```python
from build123d import *

# Parameters (mm, degrees)
SKETCH3_R          = 0.5
CUT_EXTRUDE1_DEPTH = 10
FILLET1_R          = 0.5
CHAMFER1_SIZE      = 0.2
SKETCH4_W          = 1
SKETCH4_H          = 12.5
SKETCH4_W_2        = 12.5
SKETCH4_H_2        = 1
CUT_EXTRUDE2_DEPTH = 4


with BuildPart() as part:
    # Sketch2 → Revolve1 (revolve)
    with BuildSketch(Plane(origin=(0, 0, 0), x_dir=(0, 0, -1), z_dir=(1, 0, 0)), mode=Mode.PRIVATE) as revolve1_sk:
        Polygon((0, 0), (0, 7.25), (1, 7.25), (1, 6.1), (5, 6.1), (5, 5.1), (1, 5.1), (1, 0), align=None)
    revolve(revolve1_sk.sketch.rotate(Axis((0, 0, 0), (0, 0, -1)), 90), axis=Axis((0, 0, 0), (0, 0, -1)))

    # Sketch3 → Cut-Extrude1 (cut)
    with BuildSketch(Plane.XY):
        with Locations((-1.425, 1.425)):
            Circle(SKETCH3_R)
        with Locations((1.425, 1.425)):
            Circle(SKETCH3_R)
        with Locations((0, 1.425)):
            Circle(SKETCH3_R)
        with Locations((1.425, 0)):
            Circle(SKETCH3_R)
        with Locations((1.425, -1.425)):
            Circle(SKETCH3_R)
        with Locations((0, -1.425)):
            Circle(SKETCH3_R)
        with Locations((-1.425, -1.425)):
            Circle(SKETCH3_R)
        with Locations((-1.425, 0)):
            Circle(SKETCH3_R)
        with Locations((-2.925, 2.925)):
            Circle(SKETCH3_R)
        with Locations((0, 2.925)):
            Circle(SKETCH3_R)
        with Locations((2.925, 2.925)):
            Circle(SKETCH3_R)
        with Locations((2.925, 0)):
            Circle(SKETCH3_R)
        with Locations((2.925, -2.925)):
            Circle(SKETCH3_R)
        with Locations((0, -2.925)):
            Circle(SKETCH3_R)
        with Locations((-2.925, -2.925)):
            Circle(SKETCH3_R)
        with Locations((-2.925, 0)):
            Circle(SKETCH3_R)
        with Locations((-1.425, 2.925)):
            Circle(SKETCH3_R)
        with Locations((1.425, 2.925)):
            Circle(SKETCH3_R)
        with Locations((2.925, 1.425)):
            Circle(SKETCH3_R)
        with Locations((2.925, -1.425)):
            Circle(SKETCH3_R)
        with Locations((1.425, -2.925)):
            Circle(SKETCH3_R)
        with Locations((-1.425, -2.925)):
            Circle(SKETCH3_R)
        with Locations((-2.925, -1.425)):
            Circle(SKETCH3_R)
        with Locations((-2.925, 1.425)):
            Circle(SKETCH3_R)
        with Locations((-1.425, 4.225)):
            Circle(SKETCH3_R)
        with Locations((0, 4.225)):
            Circle(SKETCH3_R)
        with Locations((1.425, 4.225)):
            Circle(SKETCH3_R)
        with Locations((4.225, 1.425)):
            Circle(SKETCH3_R)
        with Locations((4.225, 0)):
            Circle(SKETCH3_R)
        with Locations((4.225, -1.425)):
            Circle(SKETCH3_R)
        with Locations((1.425, -4.225)):
            Circle(SKETCH3_R)
        with Locations((0, -4.225)):
            Circle(SKETCH3_R)
        with Locations((-1.425, -4.225)):
            Circle(SKETCH3_R)
        with Locations((-4.225, -1.425)):
            Circle(SKETCH3_R)
        with Locations((-4.225, 0)):
            Circle(SKETCH3_R)
        with Locations((-4.225, 1.425)):
            Circle(SKETCH3_R)
        Circle(SKETCH3_R)
    extrude(amount=-CUT_EXTRUDE1_DEPTH, mode=Mode.SUBTRACT)

    # Fillet1
    fillet1_edges = [part.edges().sort_by_distance(p)[0] for p in [
        (-6.1, 0, -5),
        (-7.25, 0, 0),
    ]]
    fillet(fillet1_edges, radius=FILLET1_R)

    # Chamfer1
    chamfer1_edges = [part.edges().sort_by_distance(p)[0] for p in [
        (-5.1, 0, -5),
    ]]
    chamfer(chamfer1_edges, length=CHAMFER1_SIZE)

    # Sketch4 → Cut-Extrude2 (cut)
    with BuildSketch(Plane(origin=(0, 0, -5), x_dir=(-1, 0, 0), z_dir=(0, 0, -1))):
        Rectangle(SKETCH4_W, SKETCH4_H)
        Rectangle(SKETCH4_W_2, SKETCH4_H_2)
    extrude(amount=-CUT_EXTRUDE2_DEPTH, mode=Mode.SUBTRACT)


solid = part.part
```
Design review of the part built by this model. Coordinates are the model's own, in mm. A direction names the side the tool comes from. Give positions to 0.01 mm unless a question says otherwise; leave off trailing zeros. Order: outer loops, then holes, each group sorted by start corner. A loop starts at its lowest first (then second) coordinate and runs counter-clockwise, first axis right, second up. Notation, with made-up numbers: (7.5, 72.5) - (62.5, 72.5) arc R29 cw to (62.5, 92.5) - close; hole circle Ø8 at (74, 28). An arc over 180 degrees is marked (long way). Use a Markdown table: item, result. Add a question column.
(1) Clearance check with flat-ended pins moving along their axes: P1, Ø1.1, axis at x = 6, z = -3.5, coming from the +Y side; P2, Ø1.5, axis at y = 2, z = -2, coming from the +X side; P3, Ø1.1, axis at y = 5.5, z = -2, coming from the +X side. State where each tip first meets the part, or that it passes through.
(2) Wall thickness on probe 1 along X at (y, z) = (-2.75, -0.4); probe 2 along X at (y, z) = (-1, -4.25); probe 3 along X at (y, z) = (-1.25, -1.55): over which ranges is each line inside the solid? List them lowest first. Write a range as [from, to].
(3) Machinability: for faces 1 (the face through (5.6, 0.5, -3)), 2 (the face through (3.16, -0.44, -0.49)), which of the approach directions +Z, -Z, +X, -X, +Y, -Y give a long, thin tool a straight path to every point of the face, cutting with its end or side? Answer none if there is none.
(4) Add section A-A on x = 0. Give the number of separate pieces and of enclosed holes in the cut face, then the cut area to 3 significant figures.
(5) Add section C-C on z = -3.85. Give the boundary of the cut face in (x, y).
Report:
| question | item | result |
|---|---|---|
| 1 | P1 | stops at y = 2.74 |
| 1 | P2 | stops at x = 5.97 |
| 1 | P3 | stops at x = 3.56 |
| 2 | probe 1 | x = [-6.7, -3.39], [-2.46, -1.89], [-0.96, -0.47], [0.47, 0.96], [1.89, 2.46], [3.39, 6.7] |
| 2 | probe 2 | x = [-6.02, -5], [5, 6.02] |
| 2 | probe 3 | x = [-5.97, -4.94], [4.94, 5.97] |
| 3 | face 1 | -Z, +X, -X |
| 3 | face 2 | +Z, -Z |
| 4 | separate pieces | 8 |
| 4 | enclosed holes | 0 |
| 4 | area | 7.39 mm² |
| 5 | outline | (-6.08, -0.5) arc R6.1 ccw to (-0.5, -6.08) - (-0.5, -5.08) arc R5.1 cw to (-5.08, -0.5) - close; (-6.08, 0.5) - (-5.08, 0.5) arc R5.1 cw to (-0.5, 5.08) - (-0.5, 6.08) arc R6.1 ccw to start; (0.5, -6.08) arc R6.1 ccw to (6.08, -0.5) - (5.08, -0.5) arc R5.1 cw to (0.5, -5.08) - close; (0.5, 5.08) arc R5.1 cw to (5.08, 0.5) - (6.08, 0.5) arc R6.1 ccw to (0.5, 6.08) - close |
